Check sheet for the modelled part. Datum: model origin and axes. Units: mm. A direction names the side the tool comes from. Coordinates: 2 decimals unless noted, no trailing zeros. Write each loop counter-clockwise with the first axis right and the second up, starting at its lowest first coordinate (ties: lowest second). Pieces come first, ordered by that corner, then holes. Notation, with made-up numbers: M -24.5,82 L 4.5,82 A29 ccw 4.5,114 Z; hole C -38,-36 d2. An arc over 180 degrees is marked long. Answer as CSV lines item,"result". Start each with the question number.
1) Draft check along X on faces 1 (the flat face through (-23, 52, 6.35)), 2 (the flat face through (0, 57, 3)), 3 (the cylindrical face through (-17.15, 15.15, 3.22)). Enter one of: +X half, -X half, draft (parallel to the pull), parting line (faces both ways), or undercut.
2) Section check C-C (x = -3.5). Record the cut outline in (y, z) (3 decimals).
3) Access from +Z, -Z, +X, -X, +Y, -Y to the whole of each face (thin tool, end or side, straight path). Record for faces 4 (the flat face through (-27.7, 28.62, 3.22)), 5 (the flat face through (-23, 101.6, 3)).
4) Section check B-B (z = 4.5). Record the cut outline in (x, y) (3 decimals), and give its area (3 significant figures).
5) Section check A-A (y = 69.85). Record the cut outline in (x, z) (3 decimals), and give its area (3 significant figures).
6) Go/stop test with flat-tipped pins: pin 1 Ø6 at (x, y) = (-11.3, 28.33) entering from +Z; pin 2 Ø4.5 at (x, y) = (-22.225, 69.85) entering from -Z. Record where each tip stops, or that it passes through.
7) Material ranges on L1, parallel to Y at x = -19, z = 2.25; L2, parallel to X at y = 26.5, z = 2.5; L3, parallel to Y at x = -24.5, z = 1.75, recorded low to high. Write a range as [from, to].
from build123d import *

# Parameters (mm, degrees)
SKETCH1_W            = 44.45
SKETCH1_H            = 101.6
BOSS_EXTRUDE2_DEPTH  = 6.35
FILLET1_R            = 12.7
M5_CLEARANCE_HOLE1_D = 5.5
CUT_EXTRUDE1_DEPTH   = 112.079633597
M4_CLEARANCE_HOLE1_D = 4.5


with BuildPart() as part:
    # Sketch1 → Boss-Extrude2 (new body)
    with BuildSketch(Plane.XY):
        with Locations((-22.225, 50.8)):
            Rectangle(SKETCH1_W, SKETCH1_H)
    extrude(amount=BOSS_EXTRUDE2_DEPTH)

    # Fillet1
    fillet1_edges = [part.edges().sort_by_distance(p)[0] for p in [
        (0, 0, 3.175),
        (-44.45, 0, 3.175),
    ]]
    fillet(fillet1_edges, radius=FILLET1_R)

    # M5 Clearance Hole1 (through all)
    with Locations(Plane(origin=(0, 0, 0), x_dir=(-1, 0, 0), z_dir=(0, 0, -1))):
        with Locations((22.225, 88.9), (22.225, 69.85)):
            Hole(M5_CLEARANCE_HOLE1_D / 2)

    # Sketch14 → Cut-Extrude1 (cut, through all)
    with BuildSketch(Plane.XY.offset(6.35)):
        Polygon((-14.892651581, 25.4), (-18.558825791, 31.75), (-25.891174209, 31.75), (-29.557348419, 25.4), (-25.891174209, 19.05), (-18.558825791, 19.05), align=None)
    extrude(amount=-CUT_EXTRUDE1_DEPTH, mode=Mode.SUBTRACT)

    # M4 Clearance Hole1 (through all)
    with Locations(Plane(origin=(0, 0, 0), x_dir=(-1, 0, 0), z_dir=(0, 0, -1))):
        with Locations((11.29679677, 28.32820323), (25.15320323, 36.32820323), (33.15320323, 22.47179677), (19.29679677, 14.47179677)):
            Hole(M4_CLEARANCE_HOLE1_D / 2)


solid = part.part
Results found:
1,face 1,"draft"
1,face 2,"+X half"
1,face 3,"undercut"
2,outline,"M 3.945,0 L 101.6,0 L 101.6,6.35 L 3.945,6.35 Z"
3,face 4,"+Z, -Z"
3,face 5,"+Z, -Z, +X, -X, +Y"
4,outline,"M -44.45,12.7 A12.7 ccw -31.75,0 L -12.7,0 A12.7 ccw 0,12.7 L 0,101.6 L -44.45,101.6 Z; hole C -33.153,22.472 d4.5; hole M -29.557,25.4 L -25.891,19.05 L -18.559,19.05 L -14.893,25.4 L -18.559,31.75 L -25.891,31.75 Z; hole C -25.153,36.328 d4.5; hole C -22.225,69.85 d5.5; hole C -22.225,88.9 d5.5; hole C -19.297,14.472 d4.5; hole C -11.297,28.328 d4.5"
4,area,"4,200 mm2"
5,outline,"M -44.45,0 L -24.975,0 L -24.975,6.35 L -44.45,6.35 Z; M -19.475,0 L 0,0 L 0,6.35 L -19.475,6.35 Z"
5,area,"247 mm2"
6,pin 1,"stops at z = 6.35"
6,pin 2,"passes through"
7,L1,"y = [0, 12.24], [16.7, 19.05], [31.75, 101.6]"
7,L2,"x = [-44.45, -28.92], [-15.53, -12.61], [-9.99, 0]"
7,L3,"y = [0, 19.05], [31.75, 34.18], [38.48, 68.31], [71.39, 87.36], [90.44, 101.6]"
